Autodesk Inventor part; units mm, degrees
ref_plane "Work Plane2" through (20, 0, 0) normal (1, 0, 0) x (0, 1, 0)
ref_plane "Work Plane3" through (0, 10, 0) normal (0, 1, 0) x (-1, 0, 0)
ref_plane "XY Plane" through (0, 0, 0) normal (0, 0, 1) x (1, 0, 0)
sketch "Sketch1" plane through (0, 0, 0) normal (1, 0, 0) x (0, 1, 0)
  circle A0 centre (0, 0) radius 16
  dimension "d0" = 32
extrude "Extrusion1" add sketch "Sketch1" along normal blind 15
sketch "Sketch2" plane through (15, 0, 0) normal (1, 0, 0) x (0, 0, -1)
  circle A0 centre (0, 0) radius 17.5
  dimension "d3" = 35
extrude "Extrusion2" add sketch "Sketch2" along normal blind 10
ref_plane "Work Plane2" through (20, 0, 0) normal (1, 0, 0) x (0, 1, 0)
mirror "Mirror1" about plane through (20, 0, 0) normal (1, 0, 0) of "Extrusion1"
thread "Thread3"
thread "Thread4"
chamfer "Chamfer2" distance 0.5 angle 45 2 edges at (15, 0, 17.5) (25, 0, 17.5)
sketch "Sketch6" plane through (40, 0, 0) normal (1, 0, 0) x (0, 0, -1)
  circle A0 centre (0, 0) radius 10
  dimension "d33" = 20
extrude "Extrusion6" add sketch "Sketch6" along normal blind 10
ref_plane "Work Plane3" through (0, 10, 0) normal (0, 1, 0) x (-1, 0, 0)
sketch "Sketch8" plane through (0, 10, 0) normal (0, 1, 0) x (-1, 0, 0)
  line L0 (-50, 10) -> (-50, -10)
  line L1 (-50, 0) -> (-45, 0)
  circle A0 centre (-45, 0) radius 2.5
  point P0 (0, 0)
  dimension "d40" = 5
  dimension "d41" = 5
extrude "Extrusion8" cut sketch "Sketch8" against normal blind 30
mirror "Mirror2" about plane through (20, 0, 0) normal (1, 0, 0) of "Extrusion6", "Extrusion8"
sketch "Sketch7" plane through (50, 0, 0) normal (1, 0, 0) x (0, 0, -1)
  circle A0 centre (0, 0) radius 4
  dimension "d36" = 8
extrude "Extrusion7" cut sketch "Sketch7" against normal blind 73
chamfer "Chamfer3" distance 0.5 angle 45 2 edges at (40, -16, 0) (0, -16, 0)
fillet "Fillet3" radius 1 2 edges at (50, 0, 10) (-10, 0, 10)
thread "Thread5"
thread "Thread6"
properties part number "sprocet adaptor2"
The listing builds one solid part. Answer for the finished solid, in the listing's coordinates (mm). A direction names the side the tool comes from. Coordinates: 2 decimals unless noted, no trailing zeros. Loops run counter-clockwise (first coordinate to the right, second up) from the corner with the lowest first, then second, coordinate; pieces in that order, holes last.
1) A tool of negligible diameter and unlimited length cuts with its end or side. For faces 1 (the face through (40, -3, -10)), 2 (the face through (0, 3, -10)), 3 (the face through (50, -4, -2)), from which of +Z, -Z, +X, -X, +Y, -Y can it reach the whole face along a straight path? Write none if from no direction.
2) Find section B-B on x = 32. Write down the section's boundary in (y, z), then the cut area to 3 significant figures.
3) Determine the mould class of faces 4 (the face through (-2.615, -6.514, -0.751)), 5 (the face through (25, -10, -13)), 6 (the face through (7.65, -3.47, 15.62)) for opening direction Z: pulls with the +Z half, pulls with the -Z half, needs draft (parallel to the pull), parting line crosses it, or undercut.
4) Flat-ended cylindrical pins translate along their axes: pin 1 Ø10 at (x, y) = (39, 8) entering from +Z; pin 2 Ø12 at (x, z) = (42.5, 3) entering from +Y; pin 3 Ø1.5 at (x, z) = (29, -10.5) entering from -Y; pin 4 Ø6 at (x, y) = (15, 2) entering from +Z. Find the tip coordinate at first contact, or state that the pin passes through.
5) Find section C-C on z = 0. Give the number of separate pieces and of enclosed holes in the cut face, then the cut area to 3 significant figures.
6) Find the intervals of material crossed by L1, parallel to X at y = -5.75, z = 0; L2, parallel to X at y = 13.5, z = 5; L3, parallel to Y at x = 5.5, z = -3, in increasing order.
7) Find section A-A on x = 45. Write down the section's boundary in (y, z).
Values:
1. face 1: +X
1. face 2: -X
1. face 3: +Z, -Z, +X, +Y, -Y
2. outline: circle Ø32 at (0, 0); hole circle Ø8 at (0, 0)
2. area: 754 mm2
3. face 4: undercut
3. face 5: needs draft
3. face 6: parting line crosses it
4. pin 1: stops at z = 15.72
4. pin 2: stops at y = 16
4. pin 3: stops at y = -12.69
4. pin 4: stops at z = 17.5
5. separate pieces: 6
5. enclosed holes: 0
5. area: 1,110 mm2
6. L1: x = -10 to -7.5, -2.5 to 42.5, 47.5 to 50
6. L2: x = 0 to 40
6. L3: y = -15.72 to -2.65, 2.65 to 15.72
7. outline: (-9.68, -2.5) arc R10 ccw to (9.68, -2.5) - (3.12, -2.5) arc R4 cw to (-3.12, -2.5) - close; (-9.68, 2.5) - (-3.12, 2.5) arc R4 cw to (3.12, 2.5) - (9.68, 2.5) arc R10 ccw to start
